from build123d import *

# Parameters (mm, degrees)
SKETCH1_R           = 24.193
SKETCH1_R_2         = 20.193
BOSS_EXTRUDE1_DEPTH = 24
CUT_EXTRUDE1_DEPTH  = 24
BOSS_EXTRUDE2_START = -24
BOSS_EXTRUDE2_DEPTH = 24
SKETCH4_R           = 4
CUT_EXTRUDE2_DEPTH  = 24
BOSS_EXTRUDE4_START = -24
BOSS_EXTRUDE4_DEPTH = 24


with BuildPart() as part:
    # Sketch1 → Boss-Extrude1 (new body)
    with BuildSketch(Plane.XY):
        Circle(SKETCH1_R)
        Circle(SKETCH1_R_2, mode=Mode.SUBTRACT)
    extrude(amount=BOSS_EXTRUDE1_DEPTH)

    # Sketch2 → Cut-Extrude1 (cut)
    with BuildSketch(Plane.XY.offset(24)):
        Polygon((0, -24.193), (-5.8341998, -24.895299835), (-12.0965, -20.951752594), (0, 0), align=None)
    extrude(amount=-CUT_EXTRUDE1_DEPTH, mode=Mode.SUBTRACT)

    # Sketch3 → Boss-Extrude2 (add)
    with BuildSketch(Plane.XY.offset(24).offset(BOSS_EXTRUDE2_START)):
        with BuildLine():
            Line((-15.990029306, -35.482601784), (-12.0965, -20.951752594))
            ThreePointArc((-12.0965, -20.951752594), (-14.346719144, -19.480064138), (-16.419734671, -17.767767512))
            Line((-16.419734671, -17.767767512), (-20.819658437, -34.188506559))
            Line((-20.819658437, -34.188506559), (-15.990029306, -35.482601784))
        make_face()
        with BuildLine():
            ThreePointArc((5.336023592, -23.597205369), (2.684591171, -24.043589982), (0, -24.193))
            Line((0, -24.193), (-3.893529306, -38.72384919))
            Line((-3.893529306, -38.72384919), (0.936099826, -40.017944416))
            Line((0.936099826, -40.017944416), (5.336023592, -23.597205369))
        make_face()
    extrude(amount=BOSS_EXTRUDE2_DEPTH)

    # Sketch4 → Cut-Extrude2 (cut)
    with BuildSketch(Plane(origin=(-10.877879131, 2.914718929, 0), x_dir=(0, 0, 1), z_dir=(-0.9659258262890682, 0.2588190451025212, 0))):
        with Locations(Location((12, -30.412085563, 0), (0, 0, 270))):
            Circle(SKETCH4_R)
    extrude(amount=-CUT_EXTRUDE2_DEPTH, mode=Mode.SUBTRACT)

    # Sketch5 → Boss-Extrude4 (add)
    with BuildSketch(Plane.XY.offset(24).offset(BOSS_EXTRUDE4_START)):
        with BuildLine():
            ThreePointArc((-6.052435886, 23.423690334), (6.261609158, 23.368643515), (16.953408399, 17.259292937))
            Line((16.953408399, 17.259292937), (25.944897535, 50.81598723))
            Line((25.944897535, 50.81598723), (3.006230693, 57.231094254))
            Line((3.006230693, 57.231094254), (-6.052435886, 23.423690334))
        make_face()
    extrude(amount=BOSS_EXTRUDE4_DEPTH)


solid = part.part
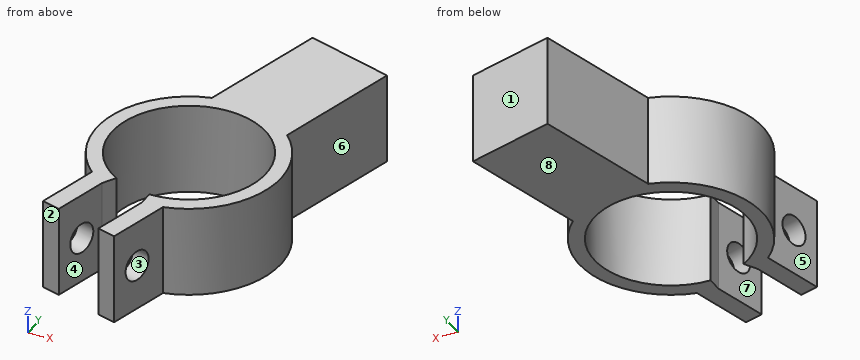
Verification items for the finished model (mm, model axes). Face numbers are marked on the shaded views. A direction names the side the tool comes from. Round coordinates to 2 decimals unless told otherwise and drop trailing zeros. Write each loop counter-clockwise with the first axis right and the second up, starting at its lowest first coordinate (ties: lowest second). Pieces come first, ordered by that corner, then holes.
(1) Section check B-B (z = 9.25). Enter the section's corners in (x, y), plus the area to 3 significant figures.
Returned:
outline: (-20.82, -34.19) - (-15.99, -35.48) - (-14.67, -30.56) - (-19.5, -29.27) - close; (-18, -23.66) - (-13.17, -24.95) - (-12.1, -20.95) - (-10.1, -17.49) arc R20.19 cw (long way) to (0, -20.19) - (0, -24.19) - (-1.07, -28.19) - (3.76, -29.48) - (5.34, -23.6) arc R24.19 ccw to (16.95, 17.26) - (25.94, 50.82) - (3.01, 57.23) - (-6.05, 23.42) arc R24.19 ccw to (-16.42, -17.77) - close; (-3.89, -38.72) - (0.94, -40.02) - (2.25, -35.1) - (-2.57, -33.8) - close
area: 1,390 mm2
(2) Depth check by flat-ended pin: pin 1 Ø6 at (y, z) = (28.5, 15.5) entering from -X; pin 2 Ø5 at (y, z) = (-20.5, 6.5) entering from -X; pin 3 Ø10 at (x, y) = (19, -18.5) entering from -Z; pin 4 Ø1 at (x, z) = (9, 3.5) entering from -Y. Enter the tip coordinate at first touch or a pass-through.
Returned:
pin 1: stops at x = -5.5
pin 2: stops at x = -17.82
pin 3: stops at z = 0
pin 4: stops at y = -22.65
(3) Section check C-C (z = 22). Enter the section's corners in (x, y), plus the area to 3 significant figures.
Returned:
outline: (-20.82, -34.19) - (-15.99, -35.48) - (-12.1, -20.95) - (-10.1, -17.49) arc R20.19 cw (long way) to (0, -20.19) - (0, -24.19) - (-3.89, -38.72) - (0.94, -40.02) - (5.34, -23.6) arc R24.19 ccw to (16.95, 17.26) - (25.94, 50.82) - (3.01, 57.23) - (-6.05, 23.42) arc R24.19 ccw to (-16.42, -17.77) - close
area: 1,450 mm2
(4) Section check D-D (x = 12). Enter the section's corners in (y, z), plus the area to 3 significant figures.
Returned:
outline: (-21.01, 0) - (-16.24, 0) - (-16.24, 24) - (-21.01, 24) - close; (16.24, 0) - (54.72, 0) - (54.72, 24) - (16.24, 24) - close
area: 1,040 mm2
(5) Material ranges on line 1 (X direction, y = 0, z = 14.25); line 2 (Y direction, x = 11, z = 10.25); line 3 (X direction, y = 10, z = 8), recorded low to high.
Returned:
line 1: x = -24.19 to -20.19, 20.19 to 24.19
line 2: y = -21.55 to -16.93, 16.93 to 55
line 3: x = -22.03 to -17.54, 17.54 to 22.03
(6) Access from +Z, -Z, +X, -X, +Y, -Y to the whole of each face (thin tool, end or side, straight path). Record for the marked faces 4, 5, 6, 7 and 8.
Returned:
face 4: +Z, -Z, -Y
face 5: +Z, -Z, -X
face 6: +Z, -Z, +X
face 7: +Z, -Z
face 8: -Z, +X, -X, +Y, -Y
(7) Mould release check, pull along Y, two halves, no side actions. Record for the marked faces 1, 2 and 3: pulls with the +Y half, pulls with the -Y half, needs draft (parallel to the pull), parting line crosses it, or undercut.
Returned:
face 1: pulls with the +Y half
face 2: pulls with the -Y half
face 3: undercut
(8) Section check A-A (y = 0). Enter the section's corners in (x, z).
Returned:
outline: (-24.19, 0) - (-20.19, 0) - (-20.19, 24) - (-24.19, 24) - close; (20.19, 0) - (24.19, 0) - (24.19, 24) - (20.19, 24) - close
